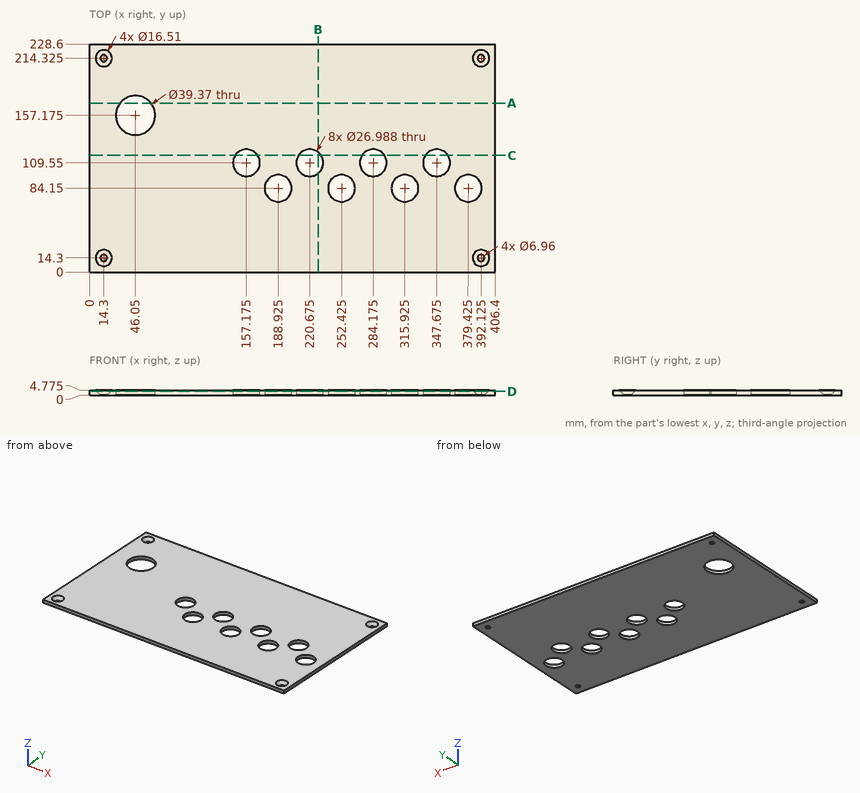
Design review of the part shown in the three views and the two pictorial views. Dimensions are in mm from the part's minimum x, y and z. Give positions to 0.01 mm unless a question says otherwise; leave off trailing zeros. Loops run counter-clockwise (first coordinate to the right, second up) from the corner with the lowest first, then second, coordinate; pieces in that order, holes last. Notation, with made-up numbers: (42, 19) -> (78, 19) arc R21 cw to (78, 33) -> close; hole circle Ø7 at (0, -23.75). An arc over 180 degrees is marked (long way). Answer as a JSON object with one key per item and string values. Group by question number.
Q1. Take a section at C-C (y = 117). Write out the cut boundary in (x, z) (1 decimal), plus the area to 3 significant figures.
Q2. Take a section at A-A (y = 169.5). Write out the cut boundary in (x, z) (1 decimal).
Q3. Take a section at B-B (x = 229). Write out the cut boundary in (y, z) (1 decimal).
Q4. Insertion check: pin 1 (21.5 mm diameter, centred on x = 252.43, y = 84.15, fed in from +Z). The pin has a flat end and moves straight along its axis. Give the tip position at first contact, or say it passes through.
Q5. Wall thickness on line 1 along X through (y, z) = (108.5, 4.4); line 2 along Y through (x, z) = (158, 4.65); line 3 along X through (y, z) = (116, 4.25): over which ranges is each line inside the solid? List them lowest first.
Q6. Take a section at D-D (z = 3.55). State how many separate pieces and enclosed holes the cut face has, plus the area to 3 significant figures.
Answer below:
{
 "1": {"outline": "(0, 0) -> (145.9, 0) -> (145.9, 4.8) -> (0, 4.8) -> close; (168.4, 0) -> (209.4, 0) -> (209.4, 4.8) -> (168.4, 4.8) -> close; (231.9, 0) -> (272.9, 0) -> (272.9, 4.8) -> (231.9, 4.8) -> close; (295.4, 0) -> (336.4, 0) -> (336.4, 4.8) -> (295.4, 4.8) -> close; (358.9, 0) -> (406.4, 0) -> (406.4, 4.8) -> (358.9, 4.8) -> close", "area": "1,510 mm2"},
 "2": {"outline": "(0, 0) -> (30.7, 0) -> (30.7, 4.8) -> (0, 4.8) -> close; (61.4, 0) -> (406.4, 0) -> (406.4, 4.8) -> (61.4, 4.8) -> close"},
 "3": {"outline": "(0, 0) -> (98.9, 0) -> (98.9, 4.8) -> (0, 4.8) -> close; (120.2, 0) -> (228.6, 0) -> (228.6, 4.8) -> (120.2, 4.8) -> close"},
 "4": {"pin 1": "passes through"},
 "5": {"line 1": "x = 0 to 143.72, 170.63 to 207.22, 234.13 to 270.72, 297.63 to 334.22, 361.13 to 406.4", "line 2": "y = 0 to 96.08, 123.02 to 228.6", "line 3": "x = 0 to 145.32, 169.03 to 208.82, 232.53 to 272.32, 296.03 to 335.82, 359.53 to 406.4"},
 "6": {"separate pieces": "1", "enclosed holes": "13", "area": "86,500 mm2"}
}
